Could you check a few things on this drawing? It's one solid part, dimensions in mm from its lowest x, y, z. Give positions to 0.01 mm unless a question says otherwise; leave off trailing zeros. Write each loop counter-clockwise with the first axis right and the second up, starting at its lowest first coordinate (ties: lowest second). Pieces come first, ordered by that corner, then holes. Notation, with made-up numbers: (55, 44.25) -> (94, 44.25) arc R18 ccw to (94, 55.25) -> close; hole circle Ø1 at (68, 19). An arc over 180 degrees is marked (long way). Use CSV: the item, a comma, the result in double quotes. Start each with the question number.
(1) Suppose I cut it at B-B on y = 48.02. List the corners of the cut face in (x, z) for me, plus the area to 4 significant figures.
(2) Suppose I cut it at A-A on x = 58. List the corners of the cut face in (y, z) for me.
(3) Suppose I cut it at C-C on y = 15. List the corners of the cut face in (x, z) for me.
(4) I need wall thicknesses on L1, parallel to Y at x = 42.76, z = 1.85; L2, parallel to X at y = 16, z = 1.15; L3, parallel to Y at x = 12.28, z = 2.45. Which ranges of each line are inside material? Lowest first, please. Write a range as [from, to].
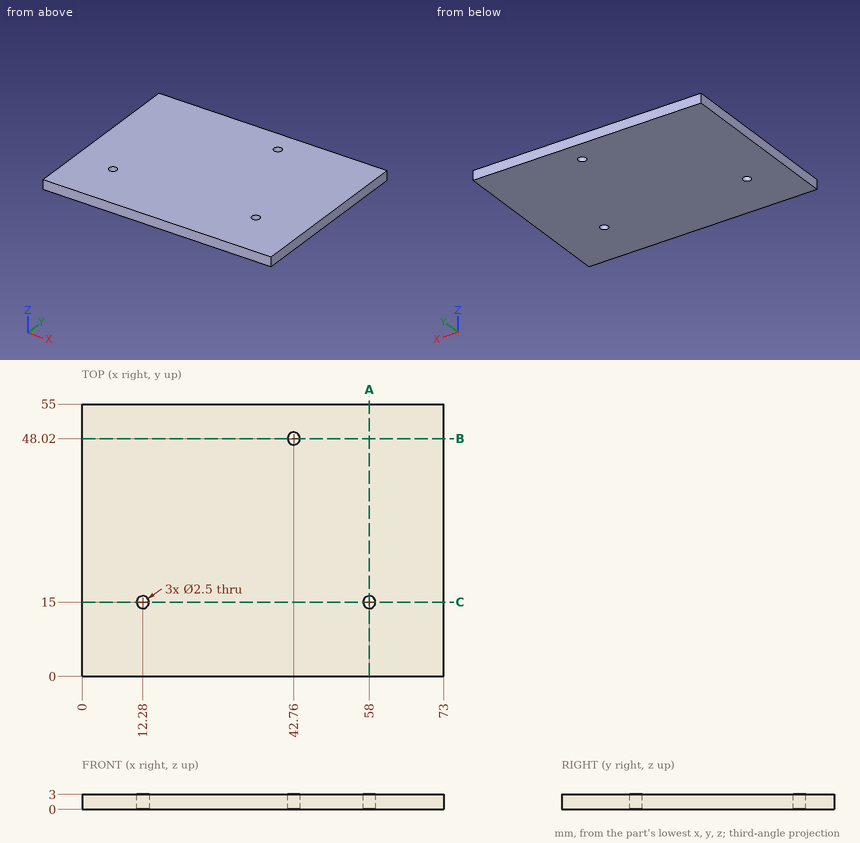
Geometry says:
1,outline,"(0, 0) -> (41.51, 0) -> (41.51, 3) -> (0, 3) -> close; (44.01, 0) -> (73, 0) -> (73, 3) -> (44.01, 3) -> close"
1,area,"211.5 mm²"
2,outline,"(0, 0) -> (13.75, 0) -> (13.75, 3) -> (0, 3) -> close; (16.25, 0) -> (55, 0) -> (55, 3) -> (16.25, 3) -> close"
3,outline,"(0, 0) -> (11.03, 0) -> (11.03, 3) -> (0, 3) -> close; (13.53, 0) -> (56.75, 0) -> (56.75, 3) -> (13.53, 3) -> close; (59.25, 0) -> (73, 0) -> (73, 3) -> (59.25, 3) -> close"
4,L1,"[0, 46.77], [49.27, 55]"
4,L2,"[0, 11.53], [13.03, 57.25], [58.75, 73]"
4,L3,"[0, 13.75], [16.25, 55]"
